from build123d import *

# Parameters (mm, degrees)
F0_R     = 2.0828
F1_DEPTH = 3.175
F2_SIZE2 = 2.4765
F2_SIZE  = 2.8448


with BuildPart() as f1:
    # F0 (on Front) → F1 (new body)
    with BuildSketch(Plane.XZ):
        with BuildLine():
            ThreePointArc((0, 6.35), (1.859872, 1.859872), (6.35, 0))
            Line((6.35, 0), (31.75, 0))
            ThreePointArc((31.75, 0), (36.240128, 1.859872), (38.1, 6.35))
            Line((38.1, 6.35), (38.1, 19.05))
            ThreePointArc((38.1, 19.05), (36.240128, 23.540128), (31.75, 25.4))
            Line((31.75, 25.4), (6.35, 25.4))
            ThreePointArc((6.35, 25.4), (1.859872, 23.540128), (0, 19.05))
            Line((0, 19.05), (0, 6.35))
        make_face()
        with Locations((19.05, 6.35)):
            Circle(F0_R, mode=Mode.SUBTRACT)
        with Locations((19.05, 19.05)):
            Circle(F0_R, mode=Mode.SUBTRACT)
    extrude(amount=F1_DEPTH)

    # F2
    f2_edges = [f1.edges().sort_by_distance(p)[0] for p in [
        (16.9672, -3.175, 19.05),
        (16.9672, -3.175, 6.35),
    ]]
    chamfer(f2_edges, length=F2_SIZE, length2=F2_SIZE2)


solid = f1.part
Input: part model. Units: mm. Frame: model coordinates. Give positions to 0.01 mm unless a question says otherwise; leave off trailing zeros. Loops run counter-clockwise (first coordinate to the right, second up) from the corner with the lowest first, then second, coordinate; pieces in that order, holes last. Notation, with made-up numbers: (-18, -14.75) - (40, -14.75) arc R24 cw to (40, 10.25) - close; hole circle Ø9 at (64.5, 79). An arc over 180 degrees is marked (long way). Use CSV: the item, a comma, the result in double quotes. Start each with the question number.
Item 1: Section A-A on x = 19.05. Return loops of the section in (y, z) (3 decimals).
Item 2: Line query: line 1 (Z direction, x = 19.05, y = -0.05); line 2 (Z direction, x = 18.5, y = -1.05); line 3 (X direction, y = -2.5, z = 8). Output: solid intervals per line, ascending.
Item 3: Section B-B on y = -1.2. Return loops of the section in (x, z).
Item 4: Section C-C on x = 2.5. Return loops of the section in (y, z) (3 decimals), then the cut area to 3 significant figures.
Item 5: Contact query for flat-ended pins moving along their axis: P1, Ø5.5, axis at x = 19.05, z = 19.05, coming from the -Y side; P2, Ø1.5, axis at x = 33, y = -1, coming from the +Z side. Output: stop coordinate, or through.
Item 6: Mould query, pull axis X, two halves, no side actions, for faces 1 (the conical face through (18.76, -0.51, 21.27)), 2 (the cylindrical face through (36.29, -1.57, 23.49)), 3 (the cylindrical face through (1.91, -1.57, 23.59)), 4 (the conical face through (21.184, -0.508, 7.022)). Classes: pulls with the +X half, pulls with the -X half, needs draft (parallel to the pull), parting line crosses it, or undercut.
Ans:
1,outline,"(-3.175, 0) - (0, 0) - (0, 4.267) - (-0.33, 4.267) - (-3.175, 1.791) - close; (-3.175, 10.909) - (-0.33, 8.433) - (0, 8.433) - (0, 16.967) - (-0.33, 16.967) - (-3.175, 14.491) - close; (-3.175, 23.609) - (-0.33, 21.133) - (0, 21.133) - (0, 25.4) - (-3.175, 25.4) - close"
2,line 1,"z = 0 to 4.27, 8.43 to 16.97, 21.13 to 25.4"
2,line 2,"z = 0 to 3.7, 9 to 16.4, 21.7 to 25.4"
2,line 3,"x = 0 to 15.44, 22.66 to 38.1"
3,outline,"(0, 6.35) arc R6.35 ccw to (6.35, 0) - (31.75, 0) arc R6.35 ccw to (38.1, 6.35) - (38.1, 19.05) arc R6.35 ccw to (31.75, 25.4) - (6.35, 25.4) arc R6.35 ccw to (0, 19.05) - close; hole circle Ø5.68 at (19.05, 6.35); hole circle Ø5.68 at (19.05, 19.05)"
4,outline,"(-3.175, 1.3) - (0, 1.3) - (0, 24.1) - (-3.175, 24.1) - close"
4,area,"72.4 mm2"
5,P1,"stops at y = -1.1"
5,P2,"stops at z = 25.38"
6,face 1,"undercut"
6,face 2,"pulls with the +X half"
6,face 3,"pulls with the -X half"
6,face 4,"undercut"
